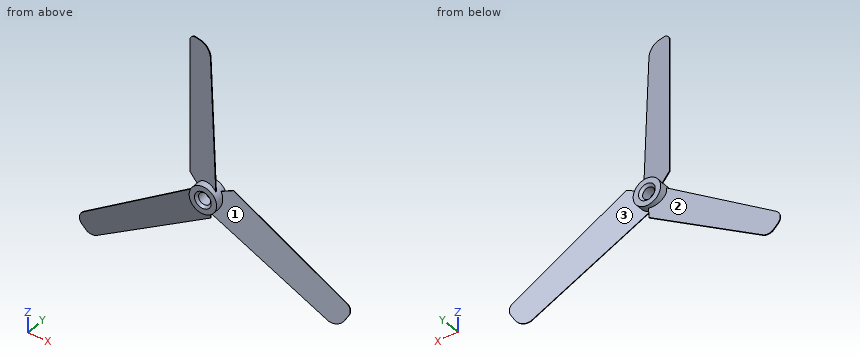
from build123d import *

# Parameters (mm, degrees)
SKETCH2_R           = 5.75
BOSS_EXTRUDE3_DEPTH = 3
BOSS_EXTRUDE4_DEPTH = 0.15
SKETCH10_R          = 2.5
CUT_EXTRUDE2_DEPTH  = 7
CIRPATTERN1_COUNT   = 3
CHAMFER1_SIZE       = 1


with BuildPart() as part:
    # Sketch2 → Boss-Extrude3 (new body, symmetric)
    with BuildSketch(Plane(origin=(0, 0, 0), x_dir=(1, 0, 0), z_dir=(0, 1, 0))):
        Circle(SKETCH2_R)
    extrude(amount=BOSS_EXTRUDE3_DEPTH, both=True)

    # Sketch7 → Boss-Extrude4 (add, symmetric)
    with BuildSketch(Plane(origin=(0, 0, 0), x_dir=(0.974370065, -0.224951054, 0), z_dir=(-0.224951054, -0.974370065, 0))):
        with BuildLine():
            Line((-4.618684487, 1.883456295), (-9.181754015, 5.498179334))
            Line((-9.181754015, 5.498179334), (-9.181754015, 60.5))
            ThreePointArc((-9.181754015, 60.5), (-8.303074359, 62.621320344), (-6.181754015, 63.5))
            Line((-6.181754015, 63.5), (-3.529096808, 63.5))
            ThreePointArc((-3.529096808, 63.5), (-0.299288732, 62.316849459), (1.401979675, 59.327335916))
            add(Edge.make_bspline(
                [(1.401979675, 59.327335916), (4.254001787, 2.228053108)],
                knots=[0, 0, 1, 1], degree=1))
            add(Edge.make_bspline(
                [(-4.618684487, 1.883456295), (-0.212236613, 8.938890212), (4.254001787, 2.228053108)],
                knots=[0, 0, 0, 1, 1, 1], degree=2))
        make_face()
    boss_extrude4 = extrude(amount=BOSS_EXTRUDE4_DEPTH, both=True)

    # Sketch10 → Cut-Extrude2 (cut, through all)
    with BuildSketch(Plane.XZ.offset(3)):
        Circle(SKETCH10_R)
    extrude(amount=-CUT_EXTRUDE2_DEPTH, mode=Mode.SUBTRACT)

    # CirPattern1: Boss-Extrude4 ×3 about axis
    cirpattern1_axis = Axis((0, 0, 0), (0, 1, 0))
    for i in range(1, CIRPATTERN1_COUNT):
        add(boss_extrude4.rotate(cirpattern1_axis, i * 360 / CIRPATTERN1_COUNT))

    # Chamfer1
    chamfer1_edges = [part.edges().sort_by_distance(p)[0] for p in [
        (-2.5, 3, 0),
        (-2.5, -3, 0),
    ]]
    chamfer(chamfer1_edges, length=CHAMFER1_SIZE)


solid = part.part
Source: CAD feature listing. Evaluate the final solid. Frame: model axes, mm. Face numbers are marked on the shaded views. Give positions to 0.01 mm unless a question says otherwise; leave off trailing zeros. Write each loop counter-clockwise with the first axis right and the second up, starting at its lowest first coordinate (ties: lowest second). Pieces come first, ordered by that corner, then holes. Notation, with made-up numbers: M 12.5,-32.75 L 49.5,-32.75 A38 ccw 49.5,6.25 Z; hole C -39.75,55 d5. An arc over 180 degrees is marked long. Return JSON: item names as keys, results as strings. Group by question number.
1) Draft query along X for the marked faces 1, 2 and 3. Return one class per face: released by +X, released by -X, zero draft, split by the parting line, or undercut.
2) Ray query, L1, parallel to Z at x = 0, y = 0.55; L2, parallel to X at y = -2.4, z = -1.5; L3, parallel to Z at x = 2, y = 2.4. Return the intervals inside material, ascending.
3) Cut plane C-C, the plane z = 24.5. Output: boundary loops of the cut face in (x, y), then the cut area to 3 significant figures.
4) First-contact query: pin 1 Ø6 at (x, z) = (0, 0) entering from -Y; pin 2 Ø3 at (y, z) = (-0.5, 43) entering from +X. Flat tips, straight axial feed; report the tip coordinate or a pass-through.
5) Cut plane A-A, the plane z = 0. Output: boundary loops of the cut face in (x, y).
6) Cut plane B-B, the plane x = -18.5. Output: boundary loops of the cut face in (y, z).
Data:
{
 "1": {"face 1": "released by +X", "face 2": "released by -X", "face 3": "undercut"},
 "2": {"L1": "z = -5.75 to -2.5, 2.5 to 5.75", "L2": "x = -5.55 to -2.48, 2.48 to 5.55", "L3": "z = -5.39 to -2.1, 2.1 to 5.39"},
 "3": {"outline": "M -8.98,1.92 L 3.03,-0.85 L 3.09,-0.56 L -8.91,2.21 Z", "area": "3.70 mm²"},
 "4": {"pin 1": "stops at y = -2.5", "pin 2": "stops at x = 2.27"},
 "5": {"outline": "M -7.91,-0.76 L -7.78,-1.05 L -5.75,-0.82 L -5.75,-3 L -3.5,-3 L -2.5,-2 L -2.5,2 L -3.5,3 L -5.75,3 L -5.75,-0.51 Z; M 2.5,-2 L 3.5,-3 L 5.75,-3 L 5.75,0.51 L 17.96,1.92 L 17.83,2.21 L 5.75,0.82 L 5.75,3 L 3.5,3 L 2.5,2 Z"},
 "6": {"outline": "M -0.91,-6.9 L 1.92,-21.05 L 2.21,-20.97 L -0.62,-6.82 Z"}
}
